Here's how the part is built. I have some questions about the finished solid (model axes, mm). A direction names the side the tool comes from. Round coordinates to 2 decimals unless told otherwise and drop trailing zeros. Loops run counter-clockwise (first coordinate to the right, second up) from the corner with the lowest first, then second, coordinate; pieces in that order, holes last. Notation, with made-up numbers: M -14,65 L 35,65 A28 ccw 35,94 Z; hole C -3,-32.5 d4. An arc over 180 degrees is marked long. One line per question, with ' | ' between items. Start each with the question number.
```python
from build123d import *

# Parameters (mm, degrees)
CUT_EXTRUDE1_DEPTH      = 26.275067654
CUT_EXTRUDE1_DEPTH_BACK = 26.275067654
SKETCH3_W               = 2.54
SKETCH3_H               = 12.7


with BuildPart() as part:
    # Sketch2 → Base-Revolve (revolve)
    with BuildSketch(Plane.XY, mode=Mode.PRIVATE) as base_revolve_sk:
        Polygon((0, 0), (0, 16.3322), (1.27, 16.3322), (1.27, 3.6322), (2.032, 1.8542), (1.27, 1.8542), (1.27, 0.531702223), (10.552917766, 0.531702223), (13.401945131, 1.801702223), (13.6398, 1.268115584), (10.795, 0), align=None)
    revolve(base_revolve_sk.sketch.rotate(Axis((0, 0, 0), (0, 1, 0)), 90), axis=Axis((0, 0, 0), (0, 1, 0)))

    # Sketch3 → Cut-Extrude1 (cut, two sides: drawn at the far end of the back side and taken through both)
    with BuildSketch(Plane.XY.offset(-CUT_EXTRUDE1_DEPTH_BACK)):
        with Locations((0, 9.9822)):
            Rectangle(SKETCH3_W, SKETCH3_H)
    extrude(amount=CUT_EXTRUDE1_DEPTH + CUT_EXTRUDE1_DEPTH_BACK, mode=Mode.SUBTRACT)


solid = part.part
```
1) I'm going to push flat-ended pins straight in: pin 1 Ø1.5 at (y, z) = (3, -6) entering from -X; pin 2 Ø2 at (x, z) = (-9, 0.5) entering from +Y; pin 3 Ø5 at (x, z) = (2, 1) entering from +Y; pin 4 Ø8 at (x, z) = (-4, -5.5) entering from +Y. Where does each tip first touch, or does it pass through?
2) We'd pull the mould along Z, two halves only. Please class faces 1 (the face through (2, 0.532, 0)), 2 (the face through (0, 0, 0)), 3 (the face through (6.653, 0.062, 8.676)): pulls with the +Z half, pulls with the -Z half, needs draft (parallel to the pull), parting line crosses it, or undercut.
3) Imagine slicing it at C-C (y = 2.65). Write out the boundary of the cut face in (x, z).
4) Imagine slicing it at B-B (x = 0). Write out the boundary of the cut face in (y, z) (3 decimals).
5) For faces 4 (the face through (-1.26, 1.18, 0.17)), 5 (the face through (9.52, 0.61, -4.95)), which set-ups out of +Z, -Z, +X, -X, +Y, -Y let a thin tool reach every point of the face, with its end or its side?
6) Imagine slicing it at A-A (z = 0). Write out the boundary of the cut face in (x, y) (3 decimals).
7) Please list where these lines run through material, in increasing order: L1, parallel to X at y = 1.7, z = -1; L2, parallel to Y at x = -1.25, z = -6.5; L3, parallel to Z at x = -3, y = 1.05. Write a range as from..to.
Results are:
1) pin 1: through | pin 2: y = 0.53 | pin 3: y = 3.63 | pin 4: y = 0.64
2) face 1: undercut | face 2: needs draft | face 3: parting line crosses it
3) outline: C 0,0 d3.38
4) outline: M 0,-10.795 L 1.268,-13.64 L 1.802,-13.402 L 0.532,-10.553 L 0.532,-1.27 L 1.854,-1.27 L 1.854,-2.032 L 3.632,-1.27 L 3.632,1.27 L 1.854,2.032 L 1.854,1.27 L 0.532,1.27 L 0.532,10.553 L 1.802,13.402 L 1.268,13.64 L 0,10.795 Z
5) face 4: none | face 5: +Y
6) outline: M -13.64,1.268 L -10.795,0 L 10.795,0 L 13.64,1.268 L 13.402,1.802 L 10.553,0.532 L 1.27,0.532 L 1.27,1.854 L 2.032,1.854 L 1.27,3.632 L -1.27,3.632 L -2.032,1.854 L -1.27,1.854 L -1.27,0.532 L -10.553,0.532 L -13.402,1.802 Z
7) L1: -13.41..-13.14, -0.78..0.78, 13.14..13.41 | L2: 0..0.53 | L3: -12.8..-11.33, 11.33..12.8
